Could you check a few things on this model? Use its own coordinates, in mm. A direction names the side the tool comes from. Round coordinates to 2 decimals unless told otherwise and drop trailing zeros. Loops run counter-clockwise (first coordinate to the right, second up) from the corner with the lowest first, then second, coordinate; pieces in that order, holes last. Notation, with made-up numbers: (-10, 51.5) -> (41, 51.5) arc R26 cw to (41, 86.5) -> close; hole circle Ø11 at (21, 42.25). An arc over 180 degrees is marked (long way). Put each result on its own line as item: value. Start each with the question number.
1. Which directions (+Z, -Z, +X, -X, +Y, -Y) give clear straight access to the entire face, cutting with the end or side of a thin tool? Please do faces 1 (the flat face through (1230.123, 1046, -5)), 2 (the cylindrical face through (1224.7, 1047.5, 7.5)), 3 (the cylindrical face through (1224.7, 1047.3, -7.5)), 4 (the flat face through (1225, 1041.877, 0)), 5 (the cylindrical face through (1189.5, 1049.82, -0.54)).
2. I need wall thicknesses on line 1 (Y direction, x = 1190, z = 0); line 2 (X direction, y = 1054.5, z = 5); line 3 (Y direction, x = 1221, z = 2.75). Which ranges of each line are inside material? Lowest first, please. Write a range as [from, to].
3. Imagine slicing it at A-A, the plane x = 1228.5. Please give me the cut outline in (y, z).
4. If we mould it in two halves opening along X, with no side actions, what happens to faces 6 (the flat face through (1247.123, 1047, 0)), 7 (the cylindrical face through (1231.137, 1043.161, 2.688)), 8 (the flat face through (1225, 1052.877, 0)), 9 (the flat face through (1232.123, 1046, -5))? For each: pulls with the +X half, pulls with the -X half, needs draft (parallel to the pull), parting line crosses it, or undercut.
5. I'm going to push flat-ended pins straight in: P1, Ø1.4, axis at x = 1243, z = -0.5, coming from the +Y side; P2, Ø8, axis at x = 1191.5, y = 1050.5, coming from the -Z side; P3, Ø2.5, axis at x = 1240.5, z = 0, coming from the -Y side; P4, Ø2, axis at x = 1235, y = 1055, coming from the -Z side. Where does each tip first touch, or does it pass through?
6. Imagine slicing it at B-B, the plane x = 1193. Please give me the cut outline in (y, z).
7. Imagine slicing it at C-C, the plane x = 1201.5. Please give me the cut outline in (y, z), and give its area (3 significant figures).
```python
from build123d import *

# Parameters (mm, degrees)
CHAMFER_1_SIZE      = 1
SKETCH_6_W          = 32.162654491
SKETCH_6_H          = 6.23657893
SKETCH_6_H_2        = 6.236578929
CUT_EXTRUDE_1_DEPTH = 25


with BuildPart() as part:
    # 草图1 → 旋转6 (revolve)
    with BuildSketch(Plane.XY, mode=Mode.PRIVATE) as revolve_6_sk:
        Polygon((1183.122729102, 1053.377429506), (1198.122729102, 1053.377429506), (1198.122729102, 1056.377429506), (1199.122729102, 1057.377429506), (1218.122729102, 1057.377429506), (1219.122729102, 1056.377429506), (1219.122729102, 1054.877429506), (1230.122729102, 1054.877429506), (1230.122729102, 1052.377429506), (1232.122729102, 1052.377429506), (1232.122729102, 1053.377429506), (1247.122729102, 1053.377429506), (1247.122729102, 1047.377429506), (1199.835322309, 1047.377429506), (1196.062603927, 1049.877429506), (1183.122729102, 1049.877429506), align=None)
    revolve(revolve_6_sk.sketch.rotate(Axis((1180.708635967, 1047.377429506, 0), (1, 0, 0)), 90), axis=Axis((1180.708635967, 1047.377429506, 0), (1, 0, 0)))

    # 倒角1
    chamfer_1_edges = [part.edges().sort_by_distance(p)[0] for p in [
        (1183.122729102, 1047.377429506, -6),
    ]]
    chamfer(chamfer_1_edges, length=CHAMFER_1_SIZE)

    # 草图6 → 拉伸1 (cut, symmetric)
    with BuildSketch(Plane.XY):
        with Locations((1235.204056347, 1055.995718971)):
            Rectangle(SKETCH_6_W, SKETCH_6_H)
        with Locations((1235.204056347, 1038.759140041)):
            Rectangle(SKETCH_6_W, SKETCH_6_H_2)
    extrude(amount=CUT_EXTRUDE_1_DEPTH, both=True, mode=Mode.SUBTRACT)


solid = part.part
```
Entries:
1. face 1: none
1. face 2: +Z, +X
1. face 3: -Z, +X
1. face 4: +Z, -Z, +X, -Y
1. face 5: -X
2. line 1: [1041.38, 1044.88], [1049.88, 1053.38]
2. line 2: [1198.12, 1219.12]
2. line 3: [1041.88, 1052.88]
3. outline: (1041.88, -5.1) arc R7.5 ccw to (1052.88, -5.1) -> (1052.88, 5.1) arc R7.5 ccw to (1041.88, 5.1) -> close
4. face 6: pulls with the +X half
4. face 7: undercut
4. face 8: needs draft
4. face 9: undercut
5. P1: y = 1052.88
5. P2: z = -6
5. P3: y = 1041.88
5. P4: through
6. outline: circle Ø12 at (1047.38, 0); hole circle Ø5 at (1047.38, 0)
7. outline: circle Ø20 at (1047.38, 0)
7. area: 314 mm^2
